from build123d import *

# Parameters (mm, degrees)
SKETCH4_R           = 1.75
SKETCH4_R_2         = 4.500000047
SKETCH4_R_3         = 5
SKETCH4_R_4         = 6
BOSS_EXTRUDE2_DEPTH = 10
SKETCH5_R           = 1.25
CUT_EXTRUDE2_DEPTH  = 15
CHAMFER1_SIZE       = 1


with BuildPart() as part:
    # Sketch4 → Boss-Extrude2 (new body)
    with BuildSketch(Plane(origin=(0, 0, 0), x_dir=(0, 0, -1), z_dir=(1, 0, 0))):
        with BuildLine():
            Line((-162.000000477, 67.500002682), (-231, 67.500002682))
            Line((-231, 67.500002682), (-231, -4.999999888))
            Line((-231, -4.999999888), (-220.999994636, -4.999999888))
            Line((-220.999994636, -4.999999888), (-206.845160655, 19.080913937))
            ThreePointArc((-206.845160655, 19.080913937), (-196.500000238, 24.999992792), (-186.154839822, 19.080913937))
            Line((-186.154839822, 19.080913937), (-172.000005841, -4.999999888))
            Line((-172.000005841, -4.999999888), (-162.000000477, -4.999999888))
            Line((-162.000000477, -4.999999888), (-162.000000477, 67.500002682))
        make_face()
        with Locations((-167.000003631, 10.000003689)):
            Circle(SKETCH4_R, mode=Mode.SUBTRACT)
        with Locations((-179.950002543, 50.158835948)):
            Circle(SKETCH4_R_2, mode=Mode.SUBTRACT)
        with Locations((-185.699998003, 36.458836819)):
            Circle(SKETCH4_R_3, mode=Mode.SUBTRACT)
        with Locations((-180.200001261, 61.499996666)):
            Circle(SKETCH4_R, mode=Mode.SUBTRACT)
        with Locations((-191.4500039, 50.158835948)):
            Circle(SKETCH4_R_2, mode=Mode.SUBTRACT)
        with Locations((-207.29999885, 36.458836819)):
            Circle(SKETCH4_R_4, mode=Mode.SUBTRACT)
        with Locations((-210.799998228, 59.499998412)):
            Circle(SKETCH4_R, mode=Mode.SUBTRACT)
        with Locations((-226, 10.000003689)):
            Circle(SKETCH4_R, mode=Mode.SUBTRACT)
    extrude(amount=-BOSS_EXTRUDE2_DEPTH)

    # Sketch5 → Cut-Extrude2 (cut)
    with BuildSketch(Plane.XY.offset(231)):
        with Locations((-5, 59.500002682)):
            Circle(SKETCH5_R)
        with Locations((-5, 31.250001397)):
            Circle(SKETCH5_R)
        with Locations((-5, 3.000002682)):
            Circle(SKETCH5_R)
    cut_extrude2 = extrude(amount=-CUT_EXTRUDE2_DEPTH, mode=Mode.SUBTRACT)

    # Mirror1: Cut-Extrude2 across plane
    add(cut_extrude2.mirror(Plane.XY.offset(196.500000238)), mode=Mode.SUBTRACT)

    # Chamfer1
    chamfer1_edges = [part.edges().sort_by_distance(p)[0] for p in [
        (0, -4.999999888, 225.999997318),
        (0, 31.250001397, 231),
        (0, 67.500002682, 196.500000238),
        (0, 31.250001397, 162.000000477),
        (-10, 31.250001397, 231),
        (-5, -4.999999888, 162.000000477),
        (-5, -4.999999888, 231),
        (-5, 67.500002682, 231),
        (-5, 67.500002682, 162.000000477),
        (-10, -4.999999888, 225.999997318),
        (-10, 7.040457024, 213.922577645),
        (-10, 24.999992792, 196.500000238),
        (-10, 7.040457024, 179.077422832),
        (-10, -4.999999888, 167.000003159),
        (-10, 31.250001397, 162.000000477),
        (0, -4.999999888, 167.000003159),
        (-10, 67.500002682, 196.500000238),
        (0, 7.040457024, 179.077422832),
        (0, 24.999992792, 196.500000238),
        (0, 7.040457024, 213.922577645),
    ]]
    chamfer(chamfer1_edges, length=CHAMFER1_SIZE)


solid = part.part
CAD build for the part. Positions are in the model's coordinates, mm. A direction names the side the tool comes from. Round coordinates to 2 decimals unless told otherwise and drop trailing zeros. Write each loop counter-clockwise with the first axis right and the second up, starting at its lowest first coordinate (ties: lowest second). Pieces come first, ordered by that corner, then holes.
(1) Mould opens along X. For faces 1 (the face through (-5, 60, 216)), 2 (the face through (-9.2, 25.2, 196.7)), 3 (the face through (-5, -5, 226)), 4 (the face through (-0.507, 7.459, 178.751)) say: pulls with the +X half, pulls with the -X half, needs draft (parallel to the pull), parting line crosses it, or undercut.
(2) Slice it at A-A, the plane z = 226. Write the cut outline in (x, y), and give its area (3 significant figures).
(3) Slice it at B-B, the plane z = 218. Write the cut outline in (x, y), and give its area (3 significant figures).
(4) Probe line 1 along Y through (x, z) = (-4.5, 179.5); line 2 along Y through (x, z) = (-5, 172.5); line 3 along Y through (x, z) = (-9, 211). List the from-to ranges inside material, lowest first.
(5) 3-axis set-ups, long thin cutter, end or side, ignore diameter. For faces 5 (the face through (-0.507, 7.122, 214.447)), 6 (the face through (-5, 30, 169)), 7 (the face through (-4.944, 7.209, 179.177)): which of +Z, -Z, +X, -X, +Y, -Y reach the whole face in a straight line?
(6) Drop flat-ended pins along their axis: P1, Ø3, axis at x = -5, y = 31.25, coming from the -Z side; P2, Ø7, axis at y = 36.46, z = 207.3, coming from the -X side; P3, Ø2, axis at x = -5, y = 3, coming from the +Z side; P4, Ø6, axis at x = -1, z = 217, coming from the -Y side. Give the stop position or say it passes through.
(7) Slice it at C-C, the plane x = -2. Count the separate pieces of the cut face and the enclosed holes in it, and give its area (3 significant figures).
From the geometry:
1. face 1: undercut
1. face 2: pulls with the -X half
1. face 3: needs draft
1. face 4: pulls with the +X half
2. outline: (-10, -4) - (-9, -5) - (-1, -5) - (0, -4) - (0, 8.25) - (-10, 8.25) - close; (-10, 11.75) - (0, 11.75) - (0, 66.5) - (-1, 67.5) - (-9, 67.5) - (-10, 66.5) - close; hole circle Ø2.5 at (-5, 3); hole circle Ø2.5 at (-5, 31.25); hole circle Ø2.5 at (-5, 59.5)
2. area: 673 mm2
3. outline: (-10, 2.08) - (-9, 0.1) - (-1, 0.1) - (0, 2.08) - (0, 66.5) - (-1, 67.5) - (-9, 67.5) - (-10, 66.5) - close; hole circle Ø2.5 at (-5, 3); hole circle Ø2.5 at (-5, 31.25); hole circle Ø2.5 at (-5, 59.5)
3. area: 656 mm2
4. line 1: y = 7.76 to 45.68, 54.64 to 59.9, 63.1 to 67.5
4. line 2: y = -4.15 to 1.75, 4.25 to 30, 32.5 to 58.25, 60.75 to 67.5
4. line 3: y = 12.01 to 31.74, 41.18 to 57.76, 61.24 to 67.5
5. face 5: +X, -Y
5. face 6: -Z
5. face 7: +X, -X, -Y
6. P1: stops at z = 162
6. P2: passes through
6. P3: stops at z = 216
6. P4: stops at y = -3.3
7. separate pieces: 1
7. enclosed holes: 8
7. area: 3,720 mm2
